```python
from build123d import *

# Parameters (mm, degrees)
SKETCH1_W           = 101.6
SKETCH1_H           = 101.6
BOSS_EXTRUDE1_DEPTH = 25.4
SKETCH2_R           = 41.91
CUT_EXTRUDE1_DEPTH  = 77.2
SKETCH3_W           = 25.4
SKETCH3_H           = 34.66394105
CUT_EXTRUDE2_DEPTH  = 77.2
SKETCH4_R           = 3.429
CUT_EXTRUDE3_DEPTH  = 77.2
SKETCH5_R           = 3.429
CUT_EXTRUDE4_DEPTH  = 117.397422652


with BuildPart() as part:
    # Sketch1 → Boss-Extrude1 (new body)
    with BuildSketch(Plane(origin=(0, 0, 0), x_dir=(1, 0, 0), z_dir=(0, 1, 0))):
        Rectangle(SKETCH1_W, SKETCH1_H)
    extrude(amount=BOSS_EXTRUDE1_DEPTH)

    # Sketch2 → Cut-Extrude1 (cut, through all)
    with BuildSketch(Plane(origin=(0, 25.4, 0), x_dir=(1, 0, 0), z_dir=(0, 1, 0))):
        with Locations(Location((0, 0, 0), (0, 0, 270))):
            Circle(SKETCH2_R)
    extrude(amount=-CUT_EXTRUDE1_DEPTH, mode=Mode.SUBTRACT)

    # Sketch3 → Cut-Extrude2 (cut, through all)
    with BuildSketch(Plane(origin=(0, 0, 0), x_dir=(1, 0, 0), z_dir=(0, 1, 0))):
        with Locations((0, 50.8)):
            Rectangle(SKETCH3_W, SKETCH3_H)
    extrude(amount=CUT_EXTRUDE2_DEPTH, mode=Mode.SUBTRACT)

    # Sketch4 → Cut-Extrude3 (cut, through all)
    with BuildSketch(Plane(origin=(0, 25.4, 0), x_dir=(1, 0, 0), z_dir=(0, 1, 0))):
        with Locations(Location((-44.45, 44.45, 0), (0, 0, 270))):
            Circle(SKETCH4_R)
        with Locations(Location((44.45, 44.45, 0), (0, 0, 270))):
            Circle(SKETCH4_R)
        with Locations(Location((44.45, -44.45, 0), (0, 0, 270))):
            Circle(SKETCH4_R)
        with Locations(Location((-44.45, -44.45, 0), (0, 0, 270))):
            Circle(SKETCH4_R)
    extrude(amount=-CUT_EXTRUDE3_DEPTH, mode=Mode.SUBTRACT)

    # Sketch5 → Cut-Extrude4 (cut, through all)
    with BuildSketch(Plane.ZY.offset(50.8)):
        with Locations((-25.4, 12.7)):
            Circle(SKETCH5_R)
        with Locations((25.4, 12.7)):
            Circle(SKETCH5_R)
    extrude(amount=-CUT_EXTRUDE4_DEPTH, mode=Mode.SUBTRACT)


solid = part.part
```
The model under review builds one solid part; all positions refer to its coordinate system, in mm. A direction names the side the tool comes from. Give positions to 0.01 mm unless a question says otherwise; leave off trailing zeros. Write each loop counter-clockwise with the first axis right and the second up, starting at its lowest first coordinate (ties: lowest second). Pieces come first, ordered by that corner, then holes. Notation, with made-up numbers: (-32, 21) -> (-18, 21) arc R14 ccw to (-18, 39) -> close; hole circle Ø3 at (14.5, 88.5). An arc over 180 degrees is marked (long way). Put each result on its own line as item: value.
(1) For pin 1 Ø4 at (y, z) = (12.7, -25.4) entering from +X, flat-tipped, find the tip position at first contact; note if it passes through.
Results are:
pin 1: through
(2) To check wall thickness, follow probe 1 along X at (y, z) = (6.75, -44.45); probe 2 along Y at (x, z) = (-36, 25); probe 3 along Z at (x, y) = (46.5, 12.7). State the ranges of each line that lie inside material, in increasing order. Write a range as from..to.
Results are:
probe 1: -50.8..-47.88, -41.02..-12.7, 12.7..41.02, 47.88..50.8
probe 2: 0..9.29, 16.11..25.4
probe 3: -50.8..-47.2, -41.7..-28.83, -21.97..21.97, 28.83..41.7, 47.2..50.8
(3) The part is to be moulded in two halves that separate along Y. For faces 3 (the flat face through (-27, 0, 34)), 4 (the cylindrical face through (-43.017, 12.851, -28.826)), 5 (the flat face through (-27, 25.4, 34)), say which applies: pulls with the +Y half, pulls with the -Y half, needs draft (parallel to the pull), parting line crosses it, or undercut.
Results are:
face 3: pulls with the -Y half
face 4: undercut
face 5: pulls with the +Y half
(4) We need section C-C, the plane z = -44.45. Give the boundary of the cut face in (x, y).
Results are:
outline: (-50.8, 0) -> (-47.88, 0) -> (-47.88, 25.4) -> (-50.8, 25.4) -> close; (-41.02, 0) -> (-12.7, 0) -> (-12.7, 25.4) -> (-41.02, 25.4) -> close; (12.7, 0) -> (41.02, 0) -> (41.02, 25.4) -> (12.7, 25.4) -> close; (47.88, 0) -> (50.8, 0) -> (50.8, 25.4) -> (47.88, 25.4) -> close
(5) We need section A-A, the plane x = 44.45. Give the boundary of the cut face in (y, z), and give its area (3 significant figures).
Results are:
outline: (0, -50.8) -> (25.4, -50.8) -> (25.4, -47.88) -> (0, -47.88) -> close; (0, -41.02) -> (25.4, -41.02) -> (25.4, 41.02) -> (0, 41.02) -> close; (0, 47.88) -> (25.4, 47.88) -> (25.4, 50.8) -> (0, 50.8) -> close; hole circle Ø6.86 at (12.7, -25.4); hole circle Ø6.86 at (12.7, 25.4)
area: 2,160 mm²
(6) Tool access review of faces 1 (the flat face through (12.7, 13, -45)), 2 (the flat face through (-50.8, 13, 1)): name each direction out of +Z, -Z, +X, -X, +Y, -Y from which nothing blocks a thin tool from reaching the whole face with its end or side.
Results are:
face 1: -Z, +Y, -Y
face 2: +Z, -Z, -X, +Y, -Y
(7) We need section D-D, the plane y = 14.75. State how many separate pieces and enclosed holes the cut face has, and give its area (3 significant figures).
Results are:
separate pieces: 5
enclosed holes: 4
area: 4,030 mm²
(8) We need section B-B, the plane y = 4.5. Give the boundary of the cut face in (x, z), and give its area (3 significant figures).
Results are:
outline: (-50.8, -50.8) -> (-12.7, -50.8) -> (-12.7, -39.94) arc R41.91 cw (long way) to (12.7, -39.94) -> (12.7, -50.8) -> (50.8, -50.8) -> (50.8, 50.8) -> (-50.8, 50.8) -> close; hole circle Ø6.86 at (-44.45, -44.45); hole circle Ø6.86 at (-44.45, 44.45); hole circle Ø6.86 at (44.45, -44.45); hole circle Ø6.86 at (44.45, 44.45)
area: 4,410 mm²
